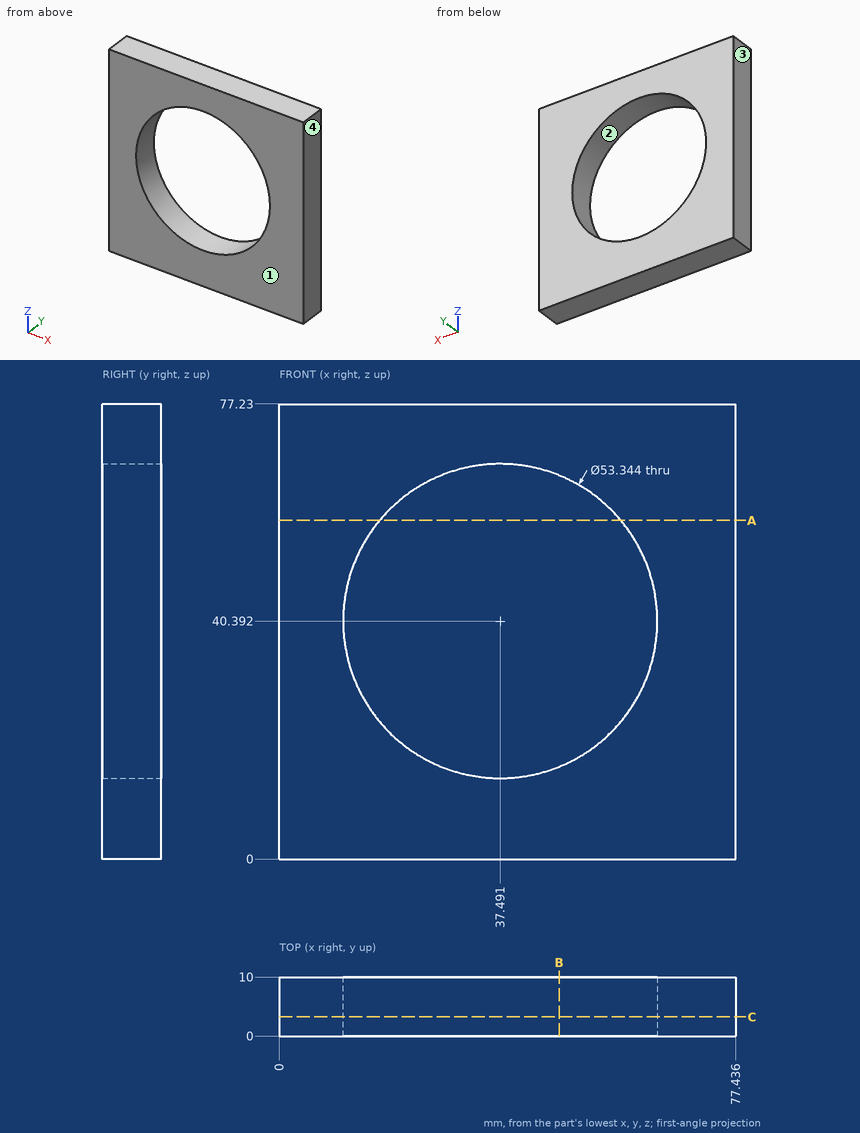
Study the drawing (mm; zero at the part's minimum x, y, z) and answer. Give positions to 0.01 mm unless a question says otherwise; leave off trailing zeros. Write each loop counter-clockwise with the first axis right and the second up, starting at its lowest first coordinate (ties: lowest second). Pieces come first, ordered by that corner, then holes. Notation, with made-up numbers: (69.25, 89.5) - (95.25, 89.5) arc R28 cw to (95.25, 111.5) - close; hole circle Ø4 at (-4.5, -15). An arc over 180 degrees is marked (long way). Write item = value, one per line. Start each with the question number.
Item 1: The mould has two halves that part along X. Classify the marked faces 1, 2, 3 and 4: +X half, -X half, draft (parallel to the pull), parting line (faces both ways), or undercut.
Item 2: This flat-tipped pin is pushed along its axis until it touches: P1, Ø12, axis at x = 34.5, z = 23.5, coming from the +Y side. Where does it stop, or does it pass through?
Item 3: Find the intervals of material crossed by probe 1 along X at (y, z) = (9, 60) (1 decimal); probe 2 along Z at (x, y) = (22.5, 7.5); probe 3 along X at (y, z) = (8.75, 63.5) (1 decimal), in increasing order. Write a range as [from, to].
Item 4: Find section B-B (x = 47.5). Give the vertices of the cut face in (y, z) (1 decimal), then the cut area to 3 significant figures.
Item 5: Find section A-A (z = 57.5). Give the vertices of the cut face in (x, y).
Item 6: Find section C-C (y = 3.25). Give the vertices of the cut face in (x, z).
Response:
q1.face_1 = draft
q1.face_2 = undercut
q1.face_3 = -X half
q1.face_4 = +X half
q2.P1 = through
q3.probe_1 = [0, 19.4], [55.6, 77.4]
q3.probe_2 = [0, 18.33], [62.45, 77.23]
q3.probe_3 = [0, 24.2], [50.8, 77.4]
q4.outline = (0, 0) - (10, 0) - (10, 15.7) - (0, 15.7) - close; (0, 65.1) - (10, 65.1) - (10, 77.2) - (0, 77.2) - close
q4.area = 278 mm²
q5.outline = (0, 0) - (17.03, 0) - (17.03, 10) - (0, 10) - close; (57.95, 0) - (77.44, 0) - (77.44, 10) - (57.95, 10) - close
q6.outline = (0, 0) - (77.44, 0) - (77.44, 77.23) - (0, 77.23) - close; hole circle Ø53.34 at (37.49, 40.39)
